Geometry: final body of the model. Coordinates: model frame, mm. A direction names the side the tool comes from. Give positions to 0.01 mm unless a question says otherwise; leave off trailing zeros. Loops run counter-clockwise (first coordinate to the right, second up) from the corner with the lowest first, then second, coordinate; pieces in that order, holes last.
```python
from build123d import *

# Parameters (mm, degrees)
SKETCH_1_R          = 2.45
EXTRUDE_1_DEPTH     = 23
SKETCH_2_OUTSIDE_W  = 16.204
SKETCH_2_OUTSIDE_H  = 16.204
CUT_EXTRUDE_1_DEPTH = 47


with BuildPart() as part:
    # 草图1 → 凸台-拉伸1 (new body, symmetric)
    with BuildSketch(Plane(origin=(0, 0, 0), x_dir=(0, 0, -1), z_dir=(1, 0, 0))):
        Circle(SKETCH_1_R)
    extrude(amount=EXTRUDE_1_DEPTH, both=True)

    # 草图2 outside → 切除-拉伸1 (cut, through all)
    with BuildSketch(Plane(origin=(23, 0, 0), x_dir=(0, 0, -1), z_dir=(1, 0, 0))):
        Rectangle(SKETCH_2_OUTSIDE_W, SKETCH_2_OUTSIDE_H)
        Polygon((-3, 0.6), (-0.6, 0.6), (-0.6, 3), (0.6, 3), (0.6, 0.6), (3, 0.6), (3, -0.6), (0.6, -0.6), (0.6, -3), (-0.6, -3), (-0.6, -0.6), (-3, -0.6), align=None, mode=Mode.SUBTRACT)
    extrude(amount=-CUT_EXTRUDE_1_DEPTH, mode=Mode.SUBTRACT)


solid = part.part
```
Q1. Pin query (flat end, axial travel): pin 1 Ø1.4 at (x, z) = (-3.5, 1.5) entering from +Y; pin 2 Ø1.4 at (x, y) = (-2.5, 1) entering from -Z; pin 3 Ø2 at (x, y) = (-13, -1.5) entering from +Z. Return the tip coordinate at first contact, or that it passes through.
Q2. Material intervals for probe 1 along Y at (x, z) = (-5, -1.7); probe 2 along Y at (x, z) = (4, -0.2), sorted ascending.
Q3. Mould query, pull axis Y, two halves, no side actions, for faces 1 (the face through (0.32, -2.45, 0.01)), 2 (the face through (-23, 0, 0)), 3 (the face through (0, 0.6, -1)). Classes: +Y half, -Y half, draft (parallel to the pull), parting line (faces both ways), or undercut.
Q4. Section query B-B, the plane z = 1.4. Return loops of the section in (x, y), and give its area (3 significant figures).
Q5. Section query A-A, the plane x = -5. Return loops of the section in (y, z).
Q6. Reachability of faces 4 (the face through (0, -2, 0.6)), 5 (the face through (0, 0.6, 2)), 6 (the face through (0, 2, -0.6)) from +Z, -Z, +X, -X, +Y, -Y: full face, straight path, thin tool, end or side. Return the list, or none.
Resolved:
1. pin 1: stops at y = 0.6
1. pin 2: stops at z = -2.43
1. pin 3: stops at z = 2.4
2. probe 1: y = -0.6 to 0.6
2. probe 2: y = -2.44 to 2.44
3. face 1: -Y half
3. face 2: draft
3. face 3: +Y half
4. outline: (-23, -0.6) - (23, -0.6) - (23, 0.6) - (-23, 0.6) - close
4. area: 55.2 mm2
5. outline: (-2.38, -0.6) - (-0.6, -0.6) - (-0.6, -2.38) arc R2.45 ccw to (0.6, -2.38) - (0.6, -0.6) - (2.38, -0.6) arc R2.45 ccw to (2.38, 0.6) - (0.6, 0.6) - (0.6, 2.38) arc R2.45 ccw to (-0.6, 2.38) - (-0.6, 0.6) - (-2.38, 0.6) arc R2.45 ccw to start
6. face 4: +Z, +X, -X, -Y
6. face 5: +Z, +X, -X, +Y
6. face 6: -Z, +X, -X, +Y
